from build123d import *

# Parameters (mm, degrees)
SKETCH1_W           = 40
SKETCH1_H           = 115
SKETCH1_R           = 6
BOSS_EXTRUDE1_DEPTH = 2
SKETCH2_R           = 2.1
CUT_EXTRUDE1_DEPTH  = 84.127913483
CUT_EXTRUDE2_DEPTH  = 84.127913483
FILLET1_R           = 1.5


with BuildPart() as part:
    # Sketch1 → Boss-Extrude1 (new body)
    with BuildSketch(Plane(origin=(0, 0, 0), x_dir=(1, 0, 0), z_dir=(0, 1, 0))):
        with Locations((-40, 0)):
            Rectangle(SKETCH1_W, SKETCH1_H)
        with Locations(Location((-40, -45, 0), (0, 0, 270))):
            Circle(SKETCH1_R, mode=Mode.SUBTRACT)
        with Locations(Location((-40, 45, 0), (0, 0, 270))):
            Circle(SKETCH1_R, mode=Mode.SUBTRACT)
    extrude(amount=BOSS_EXTRUDE1_DEPTH)

    # Sketch2 → Cut-Extrude1 (cut, through all)
    with BuildSketch(Plane(origin=(0, 2, 0), x_dir=(1, 0, 0), z_dir=(0, 1, 0))):
        with Locations(Location((-52, -32, 0), (0, 0, 270))):
            Circle(SKETCH2_R)
        with Locations(Location((-28, -32, 0), (0, 0, 90))):
            Circle(SKETCH2_R)
        with Locations(Location((-28, -50, 0), (0, 0, 270))):
            Circle(SKETCH2_R)
        with Locations(Location((-52, -50, 0), (0, 0, 90))):
            Circle(SKETCH2_R)
        with Locations(Location((-28, 50, 0), (0, 0, 90))):
            Circle(SKETCH2_R)
        with Locations(Location((-52, 50, 0), (0, 0, 270))):
            Circle(SKETCH2_R)
        with Locations(Location((-52, 32, 0), (0, 0, 90))):
            Circle(SKETCH2_R)
        with Locations(Location((-28, 32, 0), (0, 0, 270))):
            Circle(SKETCH2_R)
    extrude(amount=-CUT_EXTRUDE1_DEPTH, mode=Mode.SUBTRACT)

    # Sketch3 → Cut-Extrude2 (cut, through all)
    with BuildSketch(Plane(origin=(0, 2, 0), x_dir=(1, 0, 0), z_dir=(0, 1, 0))):
        with BuildLine():
            Line((-34, 47.5), (-34, 42.5))
            ThreePointArc((-34, 42.5), (-40, 36.5), (-46, 42.5))
            Line((-46, 42.5), (-46, 47.5))
            ThreePointArc((-46, 47.5), (-40, 53.5), (-34, 47.5))
        make_face()
    extrude(amount=-CUT_EXTRUDE2_DEPTH, mode=Mode.SUBTRACT)

    # Fillet1
    fillet1_edges = [part.edges().sort_by_distance(p)[0] for p in [
        (-20, 1, 57.5),
        (-60, 1, 57.5),
        (-60, 1, -57.5),
        (-20, 1, -57.5),
    ]]
    fillet(fillet1_edges, radius=FILLET1_R)


solid = part.part
Design review of the part built by this model. Coordinates are the model's own, in mm. A direction names the side the tool comes from. Round coordinates to 2 decimals unless told otherwise and drop trailing zeros. Loops run counter-clockwise (first coordinate to the right, second up) from the corner with the lowest first, then second, coordinate; pieces in that order, holes last. Notation, with made-up numbers: (29.5, 12) -> (38.5, 12) arc R24 cw to (38.5, 37) -> close; hole circle Ø4 at (85.5, 8.5). An arc over 180 degrees is marked (long way). Use one line per item in the form item = value. Start each with the question number.
Q1. We need section D-D on z = 45. Give the boundary of the cut face in (x, y).
Q2. Machinability: for faces 4 (the face through (-40, 1, 57.5)), 5 (the face through (-39.9, 1, -36.5)), which of the approach directions +Z, -Z, +X, -X, +Y, -Y give a long, thin tool a straight path to every point of the face, cutting with its end or side? Answer none if there is none.
Q3. We need section A-A on z = -32. Give the boundary of the cut face in (x, y).
Q4. Wall thickness on line 1 along Z through (x, y) = (-39.5, 0.6); line 2 along X through (y, z) = (1.65, -32); line 3 along X through (y, z) = (0.6, -50): over which ranges is each line inside the solid? List them lowest first. Write a range as [from, to].
Q5. We need section C-C on x = -43. Give the boundary of the cut face in (y, z).
Q6. We need section B-B on y = 0.85. State how many separate pieces and enclosed holes the cut face has, then the cut area to 3 significant figures.
Q7. Draft analysis for pull direction X (two halves, no side actions). For faces 1 (the face through (-50.137, 1.014, 49.031)), 2 (the face through (-40, 1, -57.5)), 3 (the face through (-60, 1, 1)), state which applies: +X half, -X half, draft (parallel to the pull), parting line (faces both ways), or undercut.
Calculated:
q1.outline = (-60, 0) -> (-46, 0) -> (-46, 2) -> (-60, 2) -> close; (-34, 0) -> (-20, 0) -> (-20, 2) -> (-34, 2) -> close
q2.face_4 = +Z, +X, -X, +Y, -Y
q2.face_5 = +Y, -Y
q3.outline = (-60, 0) -> (-54.1, 0) -> (-54.1, 2) -> (-60, 2) -> close; (-49.9, 0) -> (-30.1, 0) -> (-30.1, 2) -> (-49.9, 2) -> close; (-25.9, 0) -> (-20, 0) -> (-20, 2) -> (-25.9, 2) -> close
q4.line_1 = [-57.5, -53.48], [-36.52, 39.02], [50.98, 57.5]
q4.line_2 = [-60, -54.1], [-49.9, -30.1], [-25.9, -20]
q4.line_3 = [-60, -54.1], [-49.9, -45.45], [-34.55, -30.1], [-25.9, -20]
q5.outline = (0, -57.5) -> (2, -57.5) -> (2, -52.7) -> (0, -52.7) -> close; (0, -37.3) -> (2, -37.3) -> (2, 39.8) -> (0, 39.8) -> close; (0, 50.2) -> (2, 50.2) -> (2, 57.5) -> (0, 57.5) -> close
q6.separate_pieces = 1
q6.enclosed_holes = 10
q6.area = 4,200 mm²
q7.face_1 = undercut
q7.face_2 = draft
q7.face_3 = -X half
